from build123d import *

# Parameters (mm, degrees)
SKETCH_W   = 762
SKETCH_H   = 495.3
SKETCH_W_2 = 609.6
SKETCH_H_2 = 393.7
PAD_DEPTH  = 6.35


with BuildPart() as part:
    # Sketch → Pad (new body)
    with BuildSketch(Plane.XY.offset(6.35)):
        Rectangle(SKETCH_W, SKETCH_H)
        with Locations((25.4, 0)):
            Rectangle(SKETCH_W_2, SKETCH_H_2, mode=Mode.SUBTRACT)
    extrude(amount=PAD_DEPTH)


solid = part.part
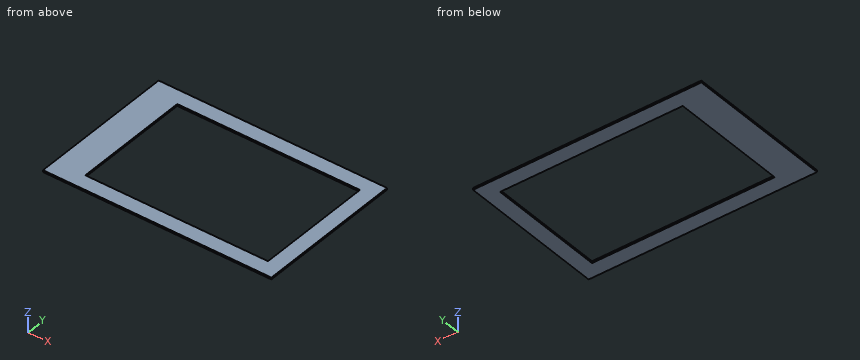
Input: part model. Units: mm. Frame: model coordinates. Give positions to 0.01 mm unless a question says otherwise; leave off trailing zeros. Loops run counter-clockwise (first coordinate to the right, second up) from the corner with the lowest first, then second, coordinate; pieces in that order, holes last. Notation, with made-up numbers: M 85.5,5.5 L 91.5,5.5 A7 cw 91.5,18.5 Z; hole C 30,66.25 d9. An arc over 180 degrees is marked long. Use CSV: the item, a comma, the result in double quotes.
(1) Section A-A, the plane y = -32.5. Return loops of the section in (x, z).
Outcome:
outline,"M -381,6.35 L -279.4,6.35 L -279.4,12.7 L -381,12.7 Z; M 330.2,6.35 L 381,6.35 L 381,12.7 L 330.2,12.7 Z"
(2) Section C-C, the plane x = 247.5. Return loops of the section in (y, z).
Outcome:
outline,"M -247.65,6.35 L -196.85,6.35 L -196.85,12.7 L -247.65,12.7 Z; M 196.85,6.35 L 247.65,6.35 L 247.65,12.7 L 196.85,12.7 Z"
(3) Section B-B, the plane z = 9.75. Return loops of the section in (x, y).
Outcome:
outline,"M -381,-247.65 L 381,-247.65 L 381,247.65 L -381,247.65 Z; hole M -279.4,-196.85 L 330.2,-196.85 L 330.2,196.85 L -279.4,196.85 Z"
(4) Material intervals for L1, parallel to X at y = -118, z = 12; L2, parallel to Y at x = 260, z = 11.25, sorted ascending. Write a range as [from, to].
Outcome:
L1,"x = [-381, -279.4], [330.2, 381]"
L2,"y = [-247.65, -196.85], [196.85, 247.65]"
